Work out the finished part from the listing and answer in its coordinate system (mm). A direction names the side the tool comes from. Coordinates: 2 decimals unless noted, no trailing zeros. Write each loop counter-clockwise with the first axis right and the second up, starting at its lowest first coordinate (ties: lowest second). Pieces come first, ordered by that corner, then holes. Notation, with made-up numbers: M 35,60 L 61,60 A16 cw 61,78 Z; hole C 28.5,57.5 d1. An arc over 180 degrees is marked long. Use CSV: the item, a comma, the result in double quotes.
Autodesk Inventor part; units mm, degrees
ref_plane "YZ Plane" through (0, 0, 0) normal (1, 0, 0) x (0, 1, 0)
ref_plane "XZ Plane" through (0, 0, 0) normal (0, 1, 0) x (-1, 0, 0)
ref_plane "XY Plane" through (0, 0, 0) normal (0, 0, 1) x (1, 0, 0)
sketch "Эскиз1" plane through (0, 0, 0) normal (0, 1, 0) x (-1, 0, 0)
  circle A0 centre (0, 0) radius 23.5
  circle A1 centre (0, 0) radius 12.5
  dimension "d0" = 47
  dimension "d1" = 25
extrude "Выдавливание1" add sketch "Эскиз1" along normal blind 6
sketch "Эскиз2" plane through (0, 6, 0) normal (0, 1, 0) x (1, 0, 0)
  circle A0 centre (0, 0) radius 13.5
  circle A1 centre (0, 0) radius 22.5
  circle A2 centre (0, 0) radius 23.5
  circle A3 centre (0, 0) radius 12.5
  dimension "d4" = 1
  dimension "d5" = 1
extrude "Выдавливание2" cut sketch "Эскиз2" against normal blind 0.5 contours A1
sketch "Эскиз3" plane through (0, 0, 0) normal (0, -1, 0) x (1, 0, 0)
  circle A0 centre (0, 0) radius 13.5
  circle A1 centre (0, 0) radius 22.5
extrude "Выдавливание3" cut sketch "Эскиз3" against normal blind 0.5
chamfer "Фаска1" distance 0.2 angle 45 8 edges at (-13.5, 0, 0) (12.5, 0, 0) (-22.5, 0, 0) (23.5, 0, 0) (23.5, 6, 0) (-22.5, 6, 0) (-13.5, 6, 0) (12.5, 6, 0)
properties part number "Подшипник 626Z" material "Титан"
Item 1: A tool of negligible diameter and unlimited length cuts with its end or side. For faces 1 (the face through (21.46, 5.65, -6.76)), 2 (the face through (-12, 0, -5)), 3 (the face through (-2.93, 0.35, -13.18)), from which of +Z, -Z, +X, -X, +Y, -Y can it reach the whole face along a straight path? Write none if from no direction.
Answer:
face 1,"+Y"
face 2,"+Z, -Z, +X, -X, -Y"
face 3,"-Y"
Item 2: The part is cut by section A-A (y = 4.85). Write down the section's boundary in (x, z), then the cut area to 3 significant figures.
Answer:
outline,"C 0,0 d47; hole C 0,0 d25"
area,"1,240 mm2"
Item 3: Given pin 1 (12 mm diameter, centred on x = 18, z = -2.5, fed in from -Y); pin 2 (1 mm diameter, centred on x = 8.5, y = 3.5, fed in from -Z); pin 3 (15 mm diameter, centred on x = 0, z = 0, fed in from -Y); pin 4 (4 mm diameter, centred on x = -17.5, z = -3.5, fed in from -Y), each flat-ended and moving along its own axis, determine where each tip first touches the part or whether it passes through.
Answer:
pin 1,"stops at y = 0"
pin 2,"stops at z = -22.1"
pin 3,"passes through"
pin 4,"stops at y = 0.5"
Item 4: Consider probe 1 along Z at (x, y) = (0, 5.7); probe 2 along Z at (x, y) = (0, 2.95); probe 3 along Y at (x, z) = (-11, 14). Determine where each line is inside the solid, lowest interval first.
Answer:
probe 1,"z = -23.5 to -22.5, -13.5 to -12.5, 12.5 to 13.5, 22.5 to 23.5"
probe 2,"z = -23.5 to -12.5, 12.5 to 23.5"
probe 3,"y = 0.5 to 5.5"
Item 5: For a pull along X with two mould halves and no side action, classify faces 4 (the face through (-12, 6, -5)), 5 (the face through (-2.93, 5.65, 13.18)), 6 (the face through (-22.4, 3, -7.1)) as released by +X, released by -X, zero draft, split by the parting line, or undercut.
Answer:
face 4,"zero draft"
face 5,"undercut"
face 6,"split by the parting line"
